```python
from build123d import *

# Parameters (mm, degrees)
F2_DEPTH = 50
F3_DEPTH = 30
F4_DEPTH = 50
F1_W     = 15
F1_H     = 60
F5_DEPTH = 50
F7_DEPTH = 15


with BuildPart() as f2:
    # F1 (on Front) → F2 (new body)
    with BuildSketch(Plane.XZ):
        Polygon((-65.4444598283, 60), (-65.4444598283, 0), (24.5555401717, 0), (24.5555401717, 29.4117647059), (-40.4444598283, 60), align=None)
    extrude(amount=-F2_DEPTH)

    # F3 (cut): a face of the model
    f3_faces = [f2.faces().sort_by_distance(p)[0] for p in [
        (-25.7092573361, 0, 25.5315584178),
    ]]
    extrude(f3_faces, amount=-F3_DEPTH, mode=Mode.SUBTRACT)

    # F1 (on Front) → F4 (join)
    with BuildSketch(Plane.XZ):
        Polygon((24.5555401717, 29.4117647059), (24.5555401717, 0), (44.5555401717, 0), (44.5555401717, 20), align=None)
    extrude(amount=-F4_DEPTH)

    # F1 (on Front) → F5 (join)
    with BuildSketch(Plane.XZ):
        with Locations((-72.9444598283, 30)):
            Rectangle(F1_W, F1_H)
    extrude(amount=-F5_DEPTH)

    # F6 (on face) → F7 (cut)
    with BuildSketch(Plane(origin=(-80.4444598283, 0, 0), x_dir=(0, -1, 0), z_dir=(-1, 0, 0))):
        Polygon((-20.1208200306, 60), (0, 50), (0, 60), align=None)
    extrude(amount=-F7_DEPTH, mode=Mode.SUBTRACT)


solid = f2.part
```
Can you work these out from the model? Positions are in its coordinate system, mm. A direction names the side the tool comes from. Give positions to 0.01 mm unless a question says otherwise; leave off trailing zeros. Order: outer loops, then holes, each group sorted by start corner. A loop starts at its lowest first (then second) coordinate and runs counter-clockwise, first axis right, second up. Notation, with made-up numbers: M 2,61.25 L 20,61.25 A24 ccw 20,72.25 Z; hole C 67.5,15 d3. An arc over 180 degrees is marked long. Write item = value, one per line. Start each with the question number.
Q1. For faces 1 (the flat face through (-31, 30, 24)), 2 (the flat face through (34, 0, 12)), which set-ups out of +Z, -Z, +X, -X, +Y, -Y let a thin tool reach every point of the face, with its end or its side?
Q2. We'd pull the mould along X, two halves only. Please class faces 3 (the flat face through (-65.444, 15, 30)), 4 (the flat face through (24.556, 15, 15)), 5 (the flat face through (-80.444, 25, 30)), 6 (the flat face through (-73.05, 10.2, 55.07)): pulls with the +X half, pulls with the -X half, needs draft (parallel to the pull), parting line crosses it, or undercut.
Q3. I need wall thicknesses on probe 1 along X at (y, z) = (15, 12.5); probe 2 along Y at (x, z) = (-61.5, 17.5); probe 3 along X at (y, z) = (7.5, 38). Which ranges of each line are inside material? Lowest first, please. Write a range as [from, to].
Q4. Suppose I cut it at D-D (x = -38.5). Write out the boundary of the cut face in (y, z).
Q5. Suppose I cut it at C-C (y = 23). Write out the boundary of the cut face in (x, z), plus the area to 3 significant figures.
Q6. Suppose I cut it at A-A (y = 7). Write out the boundary of the cut face in (x, z), plus the area to 3 significant figures.
Q7. Suppose I cut it at B-B (z = 9). Write out the boundary of the cut face in (x, y), plus the area to 3 significant figures.
Q8. Will these pins go through, and if not, where does the flat tip stop? pin 1 Ø1 at (y, z) = (15.5, 29.5) entering from +X; pin 2 Ø1 at (x, y) = (-16, 40.5) entering from -Z; pin 3 Ø3 at (y, z) = (18, 24.5) entering from +X; pin 4 Ø9 at (y, z) = (21, 39.5) entering from +X.
Check result:
q1.face_1 = +Z, -Z, -Y
q1.face_2 = +Z, -Z, +X, -X, -Y
q2.face_3 = undercut
q2.face_4 = undercut
q2.face_5 = pulls with the -X half
q2.face_6 = needs draft
q3.probe_1 = [-80.44, -65.44], [24.56, 44.56]
q3.probe_2 = [30, 50]
q3.probe_3 = [-80.44, -65.44]
q4.outline = M 30,0 L 50,0 L 50,59.08 L 30,59.08 Z
q5.outline = M -80.44,0 L -65.44,0 L -65.44,60 L -80.44,60 Z; M 24.56,0 L 44.56,0 L 44.56,20 L 24.56,29.41 Z
q5.area = 1,390 mm2
q6.outline = M -80.44,0 L -65.44,0 L -65.44,53.48 L -80.44,53.48 Z; M 24.56,0 L 44.56,0 L 44.56,20 L 24.56,29.41 Z
q6.area = 1,300 mm2
q7.outline = M -80.44,0 L -65.44,0 L -65.44,30 L 24.56,30 L 24.56,0 L 44.56,0 L 44.56,50 L -80.44,50 Z
q7.area = 3,550 mm2
q8.pin_1 = 25.43
q8.pin_2 = 0
q8.pin_3 = 38.18
q8.pin_4 = -65.44
